from build123d import *

# Parameters (mm, degrees)
F1_DEPTH = 25


with BuildPart() as f1:
    # F0 (on Front) → F1 (new body)
    with BuildSketch(Plane.XZ):
        with BuildLine():
            Line((-67.65018, -44), (-34.450579, -44))
            Line((-34.450579, -44), (-34.450579, -12))
            Line((-34.450579, -12), (-34.450579, -7.424228))
            Line((-34.450579, -7.424228), (-67.846284, -11.828058))
            ThreePointArc((-67.846284, -11.828058), (-68.778044, -12.326284), (-69.15018, -13.315183))
            Line((-69.15018, -13.315183), (-69.15018, -42.5))
            ThreePointArc((-69.15018, -42.5), (-68.71084, -43.56066), (-67.65018, -44))
        make_face()
        with BuildLine():
            Line((-34.450579, -44), (34.34982, -44))
            ThreePointArc((34.34982, -44), (35.410481, -43.56066), (35.84982, -42.5))
            Line((35.84982, -42.5), (35.84982, 7))
            ThreePointArc((35.84982, 7), (34.971141, 9.12132), (32.84982, 10))
            Line((32.84982, 10), (23.34982, 10))
            ThreePointArc((23.34982, 10), (22.28916, 9.56066), (21.84982, 8.5))
            Line((21.84982, 8.5), (21.84982, 0))
            Line((21.84982, 0), (-20.450579, -5.578075))
            Line((-20.450579, -5.578075), (-20.450579, -12))
            Line((-20.450579, -12), (-34.450579, -12))
            Line((-34.450579, -12), (-34.450579, -44))
        make_face()
    extrude(amount=F1_DEPTH)


solid = f1.part
Can you work these out from the model? Positions are in its coordinate system, mm. A direction names the side the tool comes from. Coordinates: 2 decimals unless noted, no trailing zeros. Order: outer loops, then holes, each group sorted by start corner. A loop starts at its lowest first (then second) coordinate and runs counter-clockwise, first axis right, second up. Notation, with made-up numbers: (89.5, 50) - (138.5, 50) arc R30 ccw to (138.5, 83) - close; hole circle Ø4 at (-40, -25). An arc over 180 degrees is marked (long way). Answer as a JSON object with one key per item and string values. Group by question number.
Q1. Imagine slicing it at A-A (z = -9.5). Please give me the cut outline in (x, y), and give its area (3 significant figures).
Q2. Imagine slicing it at B-B (y = -15). Please give me the cut outline in (x, z).
Q3. I need wall thicknesses on line 1 (Z direction, x = -21.5, y = -18.75); line 2 (Z direction, x = 9, y = -13.5); line 3 (X direction, y = -20.25, z = 8). Which ranges of each line are inside material? Lowest first, please. Write a range as from..to.
Q4. We'd pull the mould along X, two halves only. Please class faces 1 (the face through (-17, -12, -44)), 2 (the face through (34.99, -12.32, 9.1)), 3 (the face through (-20.451, -12, -9)): +X half, -X half, draft (parallel to the pull), parting line (faces both ways), or undercut.
Q5. Imagine slicing it at D-D (z = -2.5). Please give me the cut outline in (x, y).
Q6. Imagine slicing it at C-C (x = -8). Please give me the cut outline in (y, z), and give its area (3 significant figures).
Q7. Will these pins go through, and if not, where does the flat tip stop? P1, Ø1, axis at x = 6, y = -18.5, coming from the +Z side; P2, Ø12, axis at x = -40.5, y = -18.5, coming from the +Z side; P3, Ø7, axis at y = -16.5, z = -9, coming from the -X side.
Q8. On a 3-axis mill with a long thin cutter (end or side, diameter ignored), from which of +Z, -Z, +X, -X, +Y, -Y can I reach the whole of each face in a straight line? I mean faces 4 (the face through (-34.451, -12, -10)), 5 (the face through (21.85, -12, 4)), 6 (the face through (-17, -25, -23)). Say none if no direction works.
Determined:
{
 "1": {"outline": "(-50.19, -25) - (-34.45, -25) - (-34.45, 0) - (-50.19, 0) - close; (-20.45, -25) - (35.85, -25) - (35.85, 0) - (-20.45, 0) - close", "area": "1,800 mm2"},
 "2": {"outline": "(-69.15, -42.5) arc R1.5 ccw to (-67.65, -44) - (34.35, -44) arc R1.5 ccw to (35.85, -42.5) - (35.85, 7) arc R3 ccw to (32.85, 10) - (23.35, 10) arc R1.5 ccw to (21.85, 8.5) - (21.85, 0) - (-20.45, -5.58) - (-20.45, -12) - (-34.45, -12) - (-34.45, -7.42) - (-67.85, -11.83) arc R1.5 ccw to (-69.15, -13.32) - close"},
 "3": {"line 1": "z = -44..-12", "line 2": "z = -44..-1.69", "line 3": "x = 21.85..35.68"},
 "4": {"face 1": "draft", "face 2": "+X half", "face 3": "undercut"},
 "5": {"outline": "(2.89, -25) - (35.85, -25) - (35.85, 0) - (2.89, 0) - close"},
 "6": {"outline": "(-25, -44) - (0, -44) - (0, -3.94) - (-25, -3.94) - close", "area": "1,000 mm2"},
 "7": {"P1": "stops at z = -2.02", "P2": "stops at z = -7.43", "P3": "stops at x = -68.91"},
 "8": {"face 4": "+Z, +Y, -Y", "face 5": "+Z, -X, +Y, -Y", "face 6": "+Z, -Z, +X, -X, -Y"}
}
